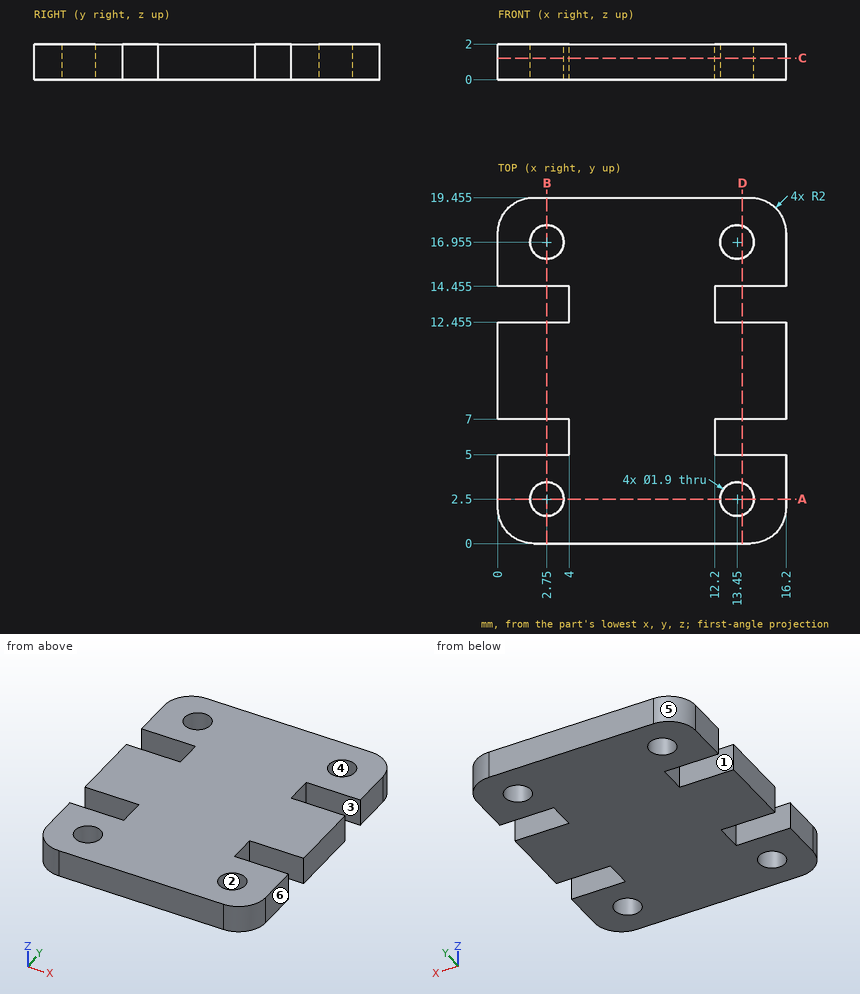
Here's the drawing with two shaded views (mm, measured from the low corner). I have some questions. A direction names the side the tool comes from. Give positions to 0.01 mm unless a question says otherwise; leave off trailing zeros. Write each loop counter-clockwise with the first axis right and the second up, starting at its lowest first coordinate (ties: lowest second). Pieces come first, ordered by that corner, then holes. Notation, with made-up numbers: (-36.75, 18.5) - (4.25, 18.5) arc R11 ccw to (4.25, 26.5) - close; hole circle Ø10 at (-36.5, 11.25). An arc over 180 degrees is marked (long way). One line per item, written item: value. Start each with the question number.
Item 1: Please list where these lines run through material, in increasing order: line 1 (Y direction, x = 3.75, z = 1.05) (3 decimals); line 2 (X direction, y = 2.5, z = 1.35); line 3 (Y direction, x = 13.45, z = 1.3) (3 decimals). Write a range as from..to.
Item 2: Imagine slicing it at B-B, the plane x = 2.75. List the corners of the cut face in (y, z) for me (3 decimals), and give its area (3 significant figures).
Item 3: Which directions (+Z, -Z, +X, -X, +Y, -Y) give clear straight access to the entire face, cutting with the end or side of a thin tool? Please do the marked faces 1, 2 and 3.
Item 4: I'm going to push a flat-ended pin straight in: pin 1 (3 mm diameter, centred on x = 13.45, y = 2.5, fed in from -Z). Where does the tip first touch, or does it pass through?
Item 5: If we mould it in two halves opening along X, with no side actions, what happens to the marked faces 4, 5 and 6? For each: +X half, -X half, draft (parallel to the pull), parting line (faces both ways), or undercut.
Item 6: Imagine slicing it at A-A, the plane y = 2.5. List the corners of the cut face in (x, z) for me, and give its area (3 significant figures).
Item 7: Imagine slicing it at D-D, the plane x = 13.75. List the corners of the cut face in (y, z) for me (3 decimals).
Item 8: Imagine slicing it at C-C, the plane z = 1.2. List the corners of the cut face in (x, y) for me (3 decimals).
Geometry says:
1. line 1: 0..5, 7..12.455, 14.455..19.455
1. line 2: 0..1.8, 3.7..12.5, 14.4..16.2
1. line 3: 0..1.55, 3.45..5, 7..12.455, 14.455..16.005, 17.905..19.455
2. outline: (0, 0) - (1.55, 0) - (1.55, 2) - (0, 2) - close; (3.45, 0) - (5, 0) - (5, 2) - (3.45, 2) - close; (7, 0) - (12.455, 0) - (12.455, 2) - (7, 2) - close; (14.455, 0) - (16.005, 0) - (16.005, 2) - (14.455, 2) - close; (17.905, 0) - (19.455, 0) - (19.455, 2) - (17.905, 2) - close
2. area: 23.3 mm^2
3. face 1: +Z, -Z, -X
3. face 2: +Z, -Z
3. face 3: +Z, -Z, +X
4. pin 1: z = 0
5. face 4: undercut
5. face 5: -X half
5. face 6: +X half
6. outline: (0, 0) - (1.8, 0) - (1.8, 2) - (0, 2) - close; (3.7, 0) - (12.5, 0) - (12.5, 2) - (3.7, 2) - close; (14.4, 0) - (16.2, 0) - (16.2, 2) - (14.4, 2) - close
6. area: 24.8 mm^2
7. outline: (0, 0) - (1.599, 0) - (1.599, 2) - (0, 2) - close; (3.401, 0) - (5, 0) - (5, 2) - (3.401, 2) - close; (7, 0) - (12.455, 0) - (12.455, 2) - (7, 2) - close; (14.455, 0) - (16.054, 0) - (16.054, 2) - (14.455, 2) - close; (17.856, 0) - (19.455, 0) - (19.455, 2) - (17.856, 2) - close
8. outline: (0, 2) arc R2 ccw to (2, 0) - (14.2, 0) arc R2 ccw to (16.2, 2) - (16.2, 5) - (12.2, 5) - (12.2, 7) - (16.2, 7) - (16.2, 12.455) - (12.2, 12.455) - (12.2, 14.455) - (16.2, 14.455) - (16.2, 17.455) arc R2 ccw to (14.2, 19.455) - (2, 19.455) arc R2 ccw to (0, 17.455) - (0, 14.455) - (4, 14.455) - (4, 12.455) - (0, 12.455) - (0, 7) - (4, 7) - (4, 5) - (0, 5) - close; hole circle Ø1.9 at (2.75, 2.5); hole circle Ø1.9 at (2.75, 16.955); hole circle Ø1.9 at (13.45, 2.5); hole circle Ø1.9 at (13.45, 16.955)
